from build123d import *

# Parameters (mm, degrees)
SKETCH1_R           = 25
BOSS_EXTRUDE1_DEPTH = 246.875
SKETCH2_R           = 100
BOSS_EXTRUDE2_DEPTH = 50
FILLET1_R           = 10
SKETCH3_R           = 40.935
BOSS_EXTRUDE3_DEPTH = 5
BOSS_EXTRUDE4_DEPTH = 25
SKETCH5_R           = 34.808926318
SKETCH5_R_2         = 26.31
CUT_EXTRUDE1_DEPTH  = 25
CUT_EXTRUDE1_TAPER  = 45


with BuildPart() as part:
    # Sketch1 → Boss-Extrude1 (new, symmetric)
    with BuildSketch(Plane.XY):
        with Locations(Location((0, 0, 0), (0, 0, 180))):
            Circle(SKETCH1_R)
    extrude(amount=BOSS_EXTRUDE1_DEPTH, both=True)

    # Sketch2 → Boss-Extrude2 (add)
    with BuildSketch(Plane.XY.offset(146.875)):
        Circle(SKETCH2_R)
    boss_extrude2 = extrude(amount=-BOSS_EXTRUDE2_DEPTH)

    # Mirror1: Boss-Extrude2 across plane
    add(boss_extrude2.mirror(Plane.XY))

    # Fillet1
    fillet1_edges = [part.edges().sort_by_distance(p)[0] for p in [
        (-100, 0, -146.875),
        (-100, 0, -96.875),
        (-100, 0, 96.875),
        (-100, 0, 146.875),
    ]]
    fillet(fillet1_edges, radius=FILLET1_R)

    # Sketch3 → Boss-Extrude3 (add)
    with BuildSketch(Plane.XY.offset(246.875)):
        Circle(SKETCH3_R)
    boss_extrude3 = extrude(amount=BOSS_EXTRUDE3_DEPTH)

    # Sketch4 → Boss-Extrude4 (add)
    with BuildSketch(Plane.XY.offset(251.875)):
        Polygon((-30.380171165, 0), (-15.190085582, -26.31), (15.190085582, -26.31), (30.380171165, 0), (15.190085582, 26.31), (-15.190085582, 26.31), align=None)
    boss_extrude4 = extrude(amount=BOSS_EXTRUDE4_DEPTH)

    # Sketch5 → Cut-Extrude1 (cut)
    with BuildSketch(Plane.XY.offset(276.875)):
        Circle(SKETCH5_R)
        Circle(SKETCH5_R_2, mode=Mode.SUBTRACT)
    cut_extrude1 = extrude(amount=-CUT_EXTRUDE1_DEPTH, taper=CUT_EXTRUDE1_TAPER, mode=Mode.SUBTRACT)

    # Mirror2: Boss-Extrude3, Boss-Extrude4, Cut-Extrude1 across plane
    add(boss_extrude3.mirror(Plane.XY))
    add(boss_extrude4.mirror(Plane.XY))
    add(cut_extrude1.mirror(Plane.XY), mode=Mode.SUBTRACT)


solid = part.part
Work out the finished part from the listing and answer in its coordinate system (mm). A direction names the side the tool comes from. Coordinates: 2 decimals unless noted, no trailing zeros. Loops run counter-clockwise (first coordinate to the right, second up) from the corner with the lowest first, then second, coordinate; pieces in that order, holes last. Notation, with made-up numbers: M 47.25,7.5 L 65.25,7.5 A20 ccw 65.25,37.5 Z; hole C 86.25,21 d4. An arc over 180 degrees is marked long. Answer in a Markdown table with one row per item. Add a question column.
1. Consider L1, parallel to Z at x = -39, y = 75 (3 decimals); L2, parallel to Z at x = 26.5, y = -2 (3 decimals); L3, parallel to Y at x = 1.5, z = 45.5. Determine where each line is inside the solid, lowest interval first.
2. A tool of negligible diameter and unlimited length cuts with its end or side. For faces 5 (the flat face through (-22.7, 13.3, -264.2)), 6 (the flat face through (19, -19, -96.875)), 7 (the flat face through (-1, -27, -251.875)), 8 (the flat face through (0, -26.31, 264)), from which of +Z, -Z, +X, -X, +Y, -Y can it reach the whole face along a straight path? Write none if from no direction.
3. Find section A-A, the plane z = 125. Write down the section's boundary in (x, y).
4. The mould has two halves that part along Z. Classify faces 1 (the conical face through (13.592, 23.675, 275.886)), 2 (the flat face through (-22.89, -12.97, 264.2)), 3 (the conical face through (13.707, -23.608, -275.886)), 4 (the flat face through (-19, -18, 246.875)): pulls with the +Z half, pulls with the -Z half, needs draft (parallel to the pull), parting line crosses it, or undercut.
5. Flat-ended cylindrical pins translate along their axes: P1, Ø5, axis at x = -57.5, y = -17.5, coming from the -Z side (3 decimals); P2, Ø12, axis at y = -17.5, z = 180, coming from the -X side; P3, Ø20, axis at x = 6.5, z = -265, coming from the +Y side. Find the tip coordinate at first contact, or state that the pin passes through.
6. Find section B-B, the plane z = -202.5. Write down the section's boundary in (x, y), then the cut area to 3 significant figures.
Reported:
| question | item | result |
|---|---|---|
| 1 | L1 | z = -146.875 to -96.875, 96.875 to 146.875 |
| 1 | L2 | z = -276.61 to -246.875, -146.875 to -96.875, 96.875 to 146.875, 246.875 to 276.61 |
| 1 | L3 | y = -24.95 to 24.95 |
| 2 | face 5 | -Z, -X, +Y |
| 2 | face 6 | none |
| 2 | face 7 | -Z |
| 2 | face 8 | +Z, +X, -X, -Y |
| 3 | outline | C 0,0 d200 |
| 4 | face 1 | pulls with the +Z half |
| 4 | face 2 | needs draft |
| 4 | face 3 | pulls with the -Z half |
| 4 | face 4 | undercut |
| 5 | P1 | stops at z = -146.875 |
| 5 | P2 | stops at x = -22.2 |
| 5 | P3 | stops at y = 26.31 |
| 6 | outline | C 0,0 d50 |
| 6 | area | 1,960 mm^2 |
